Work out the finished part from the listing and answer in its coordinate system (mm). Round coordinates to 2 decimals unless told otherwise and drop trailing zeros. Write each loop counter-clockwise with the first axis right and the second up, starting at its lowest first coordinate (ties: lowest second). Pieces come first, ordered by that corner, then holes.
1. Find section A-A (z = 0). Write down the section's boundary in (x, y), and give its area (3 significant figures).
2. Straight lines are drawn through the part: probe 1 along X at (y, z) = (1.5, 0); probe 2 along Z at (x, y) = (1, 1.05); probe 3 along Z at (x, y) = (-11, 0.15). For each, find the intervals that lie inside material, in ascending order.
3. Find section C-C (z = 11). Write down the section's boundary in (x, y), and give its area (3 significant figures).
4. Flat-ended cylindrical pins translate along their axes: pin 1 Ø1 at (x, y) = (3.5, 1) entering from +Z (3 decimals); pin 2 Ø12 at (x, z) = (7.5, -4.5) entering from -Y; pin 3 Ø1 at (y, z) = (1.5, -11) entering from -X. Find the tip coordinate at first contact, or state that the pin passes through.
5. Find section D-D (y = 0.4). Count the separate pieces of the cut face and the enclosed holes in it, and give its area (3 significant figures).
6. Find section B-B (x = 6.5). Write down the section's boundary in (y, z), and give its area (3 significant figures).
7. Determine the mould class of faces 1 (the face through (0, 2, 0)), 2 (the face through (-16.108, 0.986, -3.577)), 3 (the face through (10.48, 0.99, 3.95)) for opening direction X: pulls with the +X half, pulls with the -X half, needs draft (parallel to the pull), parting line crosses it, or undercut.
```python
from build123d import *

# Parameters (mm, degrees)
SKETCH_1_R      = 16.5
SKETCH_1_R_2    = 2.05
EXTRUDE_1_DEPTH = 2


with BuildPart() as part:
    # 草图1 → 凸台-拉伸1 (new body)
    with BuildSketch(Plane(origin=(0, 0, 0), x_dir=(1, 0, 0), z_dir=(0, 1, 0))):
        with Locations(Location((0, 0, 0), (0, 0, 270))):
            Circle(SKETCH_1_R)
        with Locations(Location((-12, 0, 0), (0, 0, 270))):
            Circle(SKETCH_1_R_2, mode=Mode.SUBTRACT)
        with Locations(Location((6, 10.392304845, 0), (0, 0, 270))):
            Circle(SKETCH_1_R_2, mode=Mode.SUBTRACT)
        with Locations(Location((6, -10.392304845, 0), (0, 0, 270))):
            Circle(SKETCH_1_R_2, mode=Mode.SUBTRACT)
        with Locations(Location((0, 12, 0), (0, 0, 270))):
            Circle(SKETCH_1_R_2, mode=Mode.SUBTRACT)
        with Locations(Location((-10.392304845, 6, 0), (0, 0, 270))):
            Circle(SKETCH_1_R_2, mode=Mode.SUBTRACT)
        with Locations(Location((10.392304845, 6, 0), (0, 0, 270))):
            Circle(SKETCH_1_R_2, mode=Mode.SUBTRACT)
        with Locations(Location((10.392304845, -6, 0), (0, 0, 270))):
            Circle(SKETCH_1_R_2, mode=Mode.SUBTRACT)
        with Locations(Location((0, -12, 0), (0, 0, 270))):
            Circle(SKETCH_1_R_2, mode=Mode.SUBTRACT)
        with Locations(Location((-10.392304845, -6, 0), (0, 0, 270))):
            Circle(SKETCH_1_R_2, mode=Mode.SUBTRACT)
    extrude(amount=EXTRUDE_1_DEPTH)


solid = part.part
```
Worked answers:
1. outline: (-16.5, 0) - (-14.05, 0) - (-14.05, 2) - (-16.5, 2) - close; (-9.95, 0) - (16.5, 0) - (16.5, 2) - (-9.95, 2) - close
1. area: 57.8 mm2
2. probe 1: x = -16.5 to -14.05, -9.95 to 16.5
2. probe 2: z = -16.47 to -13.79, -10.21 to 10.21, 13.79 to 16.47
2. probe 3: z = -12.3 to -7.96, -4.04 to -1.79, 1.79 to 4.04, 7.96 to 12.3
3. outline: (-12.3, 0) - (-1.79, 0) - (-1.79, 2) - (-12.3, 2) - close; (1.79, 0) - (4.04, 0) - (4.04, 2) - (1.79, 2) - close; (7.96, 0) - (12.3, 0) - (12.3, 2) - (7.96, 2) - close
3. area: 34.2 mm2
4. pin 1: stops at z = 16.225
4. pin 2: stops at y = 0
4. pin 3: stops at x = -12.73
5. separate pieces: 1
5. enclosed holes: 9
5. area: 736 mm2
6. outline: (0, -15.17) - (2, -15.17) - (2, -12.38) - (0, -12.38) - close; (0, -8.4) - (2, -8.4) - (2, 8.4) - (0, 8.4) - close; (0, 12.38) - (2, 12.38) - (2, 15.17) - (0, 15.17) - close
6. area: 44.8 mm2
7. face 1: needs draft
7. face 2: parting line crosses it
7. face 3: undercut
